Geometry: final body of the model. Coordinates: model frame, mm. A direction names the side the tool comes from. Give positions to 0.01 mm unless a question says otherwise; leave off trailing zeros. Write each loop counter-clockwise with the first axis right and the second up, starting at its lowest first coordinate (ties: lowest second). Pieces come first, ordered by that corner, then holes. Notation, with made-up numbers: M -40,18.25 L 2,18.25 A15 ccw 2,33.25 Z; hole C 35.25,-35.75 d5. An arc over 180 degrees is marked long. Use a Markdown table: item, result. Add a question column.
(1) Cut plane C-C (y = 3.7). Output: boundary loops of the cut face in (x, z).
(2) Draft query along X for faces 1 (the flat face through (1.2, 5, -1.2)), 2 (the cylindrical face through (-4.88, 2.46, -1.08)), 3 (the cylindrical face through (2.5, 2.5, 0)). Return one class per face: released by +X, released by -X, zero draft, split by the parting line, or undercut.
(3) Cut plane A-A (x = 0). Output: boundary loops of the cut face in (y, z).
(4) Reachability of faces 4 (the flat face through (-1, 2, -2)), 5 (the flat face through (1.2, 0, -1.2)) from +Z, -Z, +X, -X, +Y, -Y: full face, straight path, thin tool, end or side. Return the list, or none.
(5) Cut plane B-B (z = 0). Output: boundary loops of the cut face in (x, y), plus the area to 3 significant figures.
(6) Cut plane D-D (x = -4). Output: boundary loops of the cut face in (y, z), plus the area to 3 significant figures.
(7) Material intervals for L1, parallel to X at y = 3.55, z = 0.25; L2, parallel to Z at x = -1.75, y = 2.4; L3, parallel to X at y = 4.25, z = 3, sorted ascending.
(8) Pin query (flat end, axial travel): pin 1 Ø1 at (y, z) = (3, -1.5) entering from +X; pin 2 Ø1.4 at (x, y) = (2, 2) entering from -Z; pin 3 Ø1.5 at (x, y) = (3, 2.5) entering from +Z. Return the tip coordinate at first contact, or that it passes through.
```python
from build123d import *

# Parameters (mm, degrees)
SKETCH1_R           = 5
BOSS_EXTRUDE1_DEPTH = 5


with BuildPart() as part:
    # Sketch1 → Boss-Extrude1 (new body)
    with BuildSketch(Plane(origin=(0, 0, 0), x_dir=(1, 0, 0), z_dir=(0, 1, 0))):
        with Locations(Location((0, 0, 0), (0, 0, 270))):
            Circle(SKETCH1_R)
        with BuildLine():
            Line((1, -1), (1, -2.291287847))
            ThreePointArc((1, -2.291287847), (-0.289330525, -2.483201129), (-1.5, -2))
            Line((-1.5, -2), (-1.5, -1))
            Line((-1.5, -1), (-2.291287847, -1))
            ThreePointArc((-2.291287847, -1), (-2.5, 0), (-2.291287847, 1))
            Line((-2.291287847, 1), (-1, 1))
            Line((-1, 1), (-1, 2.291287847))
            ThreePointArc((-1, 2.291287847), (0, 2.5), (1, 2.291287847))
            Line((1, 2.291287847), (1, 1))
            Line((1, 1), (2.291287847, 1))
            ThreePointArc((2.291287847, 1), (2.5, 0), (2.291287847, -1))
            Line((2.291287847, -1), (1, -1))
        make_face(mode=Mode.SUBTRACT)
    extrude(amount=BOSS_EXTRUDE1_DEPTH)


solid = part.part
```
Answer list:
| question | item | result |
|---|---|---|
| 1 | outline | C 0,0 d10; hole M -2.29,-1 L -1,-1 L -1,-2.29 A2.5 ccw 1,-2.29 L 1,-1 L 2.29,-1 A2.5 ccw 2.29,1 L 1,1 L 1,2.29 A2.5 ccw -1.5,2 L -1.5,1 L -2.29,1 A2.5 ccw Z |
| 2 | face 1 | zero draft |
| 2 | face 2 | split by the parting line |
| 2 | face 3 | undercut |
| 3 | outline | M 0,-5 L 5,-5 L 5,-2.5 L 0,-2.5 Z; M 0,2.5 L 5,2.5 L 5,5 L 0,5 Z |
| 4 | face 4 | +Y, -Y |
| 4 | face 5 | +Z, -Z, +X, -X, -Y |
| 5 | outline | M -5,0 L -2.5,0 L -2.5,5 L -5,5 Z; M 2.5,0 L 5,0 L 5,5 L 2.5,5 Z |
| 5 | area | 25.0 mm² |
| 6 | outline | M 0,-3 L 5,-3 L 5,3 L 0,3 Z |
| 6 | area | 30.0 mm² |
| 7 | L1 | -4.99 to -2.49, 2.49 to 4.99 |
| 7 | L2 | -4.68 to -1, 1 to 4.68 |
| 7 | L3 | -4 to 4 |
| 8 | pin 1 | x = 4.9 |
| 8 | pin 2 | z = -4.83 |
| 8 | pin 3 | z = 4.47 |
